```python
from build123d import *

# Parameters (mm, degrees)
F0_R     = 12.5
F1_DEPTH = 5
F2_W     = 10.5
F2_H     = 5.25
F3_DEPTH = 5


with BuildPart() as f1:
    # F0 (on Top) → F1 (new body)
    with BuildSketch(Plane.XY):
        Circle(F0_R)
    extrude(amount=F1_DEPTH)


with BuildPart() as f3:
    # F2 (on face) → F3 (new body)
    with BuildSketch(Plane.XY.offset(5)):
        with Locations((0, 5.625)):
            Rectangle(F2_W, F2_H)
        with Locations((0, -5.625)):
            Rectangle(F2_W, F2_H)
    extrude(amount=-F3_DEPTH)


with BuildPart() as f1_1:
    add(f1.part)

    # F4: cut F3
    add(f3.part, mode=Mode.SUBTRACT)


solid = f1_1.part
```
Verification items for the finished model (mm, model axes). A direction names the side the tool comes from. Coordinates: 2 decimals unless noted, no trailing zeros. Order: outer loops, then holes, each group sorted by start corner. A loop starts at its lowest first (then second) coordinate and runs counter-clockwise, first axis right, second up. Notation, with made-up numbers: (8, 69.25) -> (44, 69.25) arc R32 cw to (44, 97.25) -> close; hole circle Ø3 at (-25.5, 9.25). An arc over 180 degrees is marked (long way). Put each result on its own line as item: value. Start each with the question number.
1) Cross-section at A-A (x = 0). Enter the section's corners in (y, z), plus the area to 3 significant figures.
2) Cross-section at C-C (z = 4.05). Enter the section's corners in (x, y).
3) Cross-section at D-D (x = 3). Enter the section's corners in (y, z), plus the area to 3 significant figures.
4) Material ranges on L1, parallel to Y at x = 3.25, z = 4.45; L2, parallel to Y at x = -2, z = 2.6; L3, parallel to X at y = -6.5, z = 2.3, recorded low to high.
5) Go/stop test with flat-tipped pins: pin 1 (2.5 mm diameter, centred on x = 1, z = 2.5, fed in from +Y); pin 2 (2.5 mm diameter, centred on x = 1.5, z = 3, fed in from -Y); pin 3 (2.5 mm diameter, centred on y = -6, z = 1.5, fed in from -X); pin 4 (1.5 mm diameter, centred on y = 6.5, z = 2, fed in from -X). Record where each tip stops, or that it passes through.
6) Tool access check on faces 4 (the flat face through (0, 0, 0)), 5 (the flat face through (-5.25, 6, 3)). Record the directions out of +Z, -Z, +X, -X, +Y, -Y that give a thin tool (end or side, any length) a straight path to the whole face; none if there is none.
7) Release check for a two-part mould opening along Y. For faces 1 (the flat face through (0, 3, 3)), 2 (the flat face through (0, 0, 5)), 3 (the cylindrical face through (11.923, 3.755, 2.465)) record: pulls with the +Y half, pulls with the -Y half, needs draft (parallel to the pull), parting line crosses it, or undercut.
8) Cross-section at B-B (y = 5.5). Enter the section's corners in (x, z), plus the area to 3 significant figures.
Geometry check:
1. outline: (-12.5, 0) -> (-8.25, 0) -> (-8.25, 5) -> (-12.5, 5) -> close; (-3, 0) -> (3, 0) -> (3, 5) -> (-3, 5) -> close; (8.25, 0) -> (12.5, 0) -> (12.5, 5) -> (8.25, 5) -> close
1. area: 72.5 mm^2
2. outline: circle Ø25 at (0, 0); hole (-5.25, -8.25) -> (5.25, -8.25) -> (5.25, -3) -> (-5.25, -3) -> close; hole (-5.25, 3) -> (5.25, 3) -> (5.25, 8.25) -> (-5.25, 8.25) -> close
3. outline: (-12.13, 0) -> (-8.25, 0) -> (-8.25, 5) -> (-12.13, 5) -> close; (-3, 0) -> (3, 0) -> (3, 5) -> (-3, 5) -> close; (8.25, 0) -> (12.13, 0) -> (12.13, 5) -> (8.25, 5) -> close
3. area: 68.8 mm^2
4. L1: y = -12.07 to -8.25, -3 to 3, 8.25 to 12.07
4. L2: y = -12.34 to -8.25, -3 to 3, 8.25 to 12.34
4. L3: x = -10.68 to -5.25, 5.25 to 10.68
5. pin 1: stops at y = 12.5
5. pin 2: stops at y = -12.5
5. pin 3: stops at x = -11.56
5. pin 4: stops at x = -11.1
6. face 4: -Z, +X, -X, +Y, -Y
6. face 5: +Z, -Z
7. face 1: undercut
7. face 2: needs draft
7. face 3: parting line crosses it
8. outline: (-11.22, 0) -> (-5.25, 0) -> (-5.25, 5) -> (-11.22, 5) -> close; (5.25, 0) -> (11.22, 0) -> (11.22, 5) -> (5.25, 5) -> close
8. area: 59.7 mm^2
